```python
from build123d import *

# Parameters (mm, degrees)
SKETCH_2_W          = 62.35
SKETCH_2_H          = 3.8
SKETCH_2_R          = 0.5
EXTRUDE_1_DEPTH     = 2
CUT_EXTRUDE_1_REACH = 33.297
SKETCH_3_R          = 0.375


with BuildPart() as part:
    # 草图2 → 凸台-拉伸1 (new body)
    with BuildSketch(Plane.XY):
        Rectangle(SKETCH_2_W, SKETCH_2_H)
        with Locations((7.7, 0)):
            Circle(SKETCH_2_R, mode=Mode.SUBTRACT)
        with Locations((-8.3, 0)):
            Circle(SKETCH_2_R, mode=Mode.SUBTRACT)
    extrude(amount=EXTRUDE_1_DEPTH)

    # 草图3 → 切除-拉伸1 (cut, up to next)
    with BuildSketch(Plane(origin=(0, 0, 0), x_dir=(-1, 0, 0), z_dir=(0, 0, -1)), mode=Mode.PRIVATE) as cut_extrude_1_sk1:
        with Locations((29.175, 0)):
            Circle(SKETCH_3_R)
    cut_extrude_1_tool1 = extrude(cut_extrude_1_sk1.sketch, amount=-CUT_EXTRUDE_1_REACH, mode=Mode.PRIVATE) & part.part
    # 草图3 → 切除-拉伸1 (cut, up to next)
    with BuildSketch(Plane(origin=(0, 0, 0), x_dir=(-1, 0, 0), z_dir=(0, 0, -1)), mode=Mode.PRIVATE) as cut_extrude_1_sk2:
        with Locations((-29.175, 0)):
            Circle(SKETCH_3_R)
    cut_extrude_1_tool2 = extrude(cut_extrude_1_sk2.sketch, amount=-CUT_EXTRUDE_1_REACH, mode=Mode.PRIVATE) & part.part
    add(cut_extrude_1_tool1.solids().sort_by_distance((-29.175, 0, 0))[0], mode=Mode.SUBTRACT)
    add(cut_extrude_1_tool2.solids().sort_by_distance((29.175, 0, 0))[0], mode=Mode.SUBTRACT)


solid = part.part
```
Here's how the part is built. I have some questions about the finished solid (model axes, mm). Give positions to 0.01 mm unless a question says otherwise; leave off trailing zeros. Write each loop counter-clockwise with the first axis right and the second up, starting at its lowest first coordinate (ties: lowest second). Pieces come first, ordered by that corner, then holes. Notation, with made-up numbers: (61, 65.25) -> (96, 65.25) arc R32 ccw to (96, 97.25) -> close; hole circle Ø9 at (20, 81.25). An arc over 180 degrees is marked (long way). Write each question's results on one line, items separated by ' | '.
Item 1: Suppose I cut it at A-A on x = 7.7. Write out the boundary of the cut face in (y, z).
Output:
outline: (-1.9, 0) -> (-0.5, 0) -> (-0.5, 2) -> (-1.9, 2) -> close; (0.5, 0) -> (1.9, 0) -> (1.9, 2) -> (0.5, 2) -> close
Item 2: We'd pull the mould along Y, two halves only. Please class faces 1 (the face through (0, 1.9, 1)), 2 (the face through (7.2, 0, 1)), 3 (the face through (31.175, 0, 1)): pulls with the +Y half, pulls with the -Y half, needs draft (parallel to the pull), parting line crosses it, or undercut.
Output:
face 1: pulls with the +Y half | face 2: undercut | face 3: needs draft
Item 3: If I drill on L1, parallel to X at y = -0.05, z = 0.65 (1 decimal); L2, parallel to X at y = 0.2, z = 0.4 (3 decimals); L3, parallel to Y at x = -8.3, z = 1.1, over which ranges is the centre line in solid material (lowest first)?
Output:
L1: x = -31.2 to -29.5, -28.8 to -8.8, -7.8 to 7.2, 8.2 to 28.8, 29.5 to 31.2 | L2: x = -31.175 to -29.492, -28.858 to -8.758, -7.842 to 7.242, 8.158 to 28.858, 29.492 to 31.175 | L3: y = -1.9 to -0.5, 0.5 to 1.9
